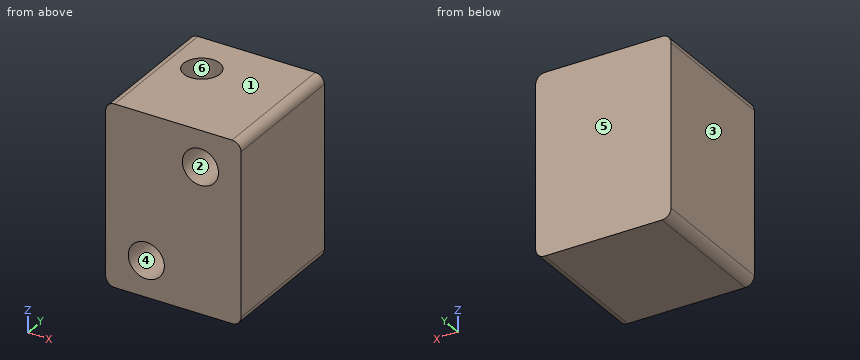
```python
from build123d import *

# Parameters (mm, degrees)
BOSS_EXTRU_1_DEPTH      = 15
ESQUISSE2_R             = 2
ENL_V_MAT_EXTRU_1_DEPTH = 12
ESQUISSE3_R             = 2
ENL_V_MAT_EXTRU_2_DEPTH = 12
CONG_1_R                = 1


with BuildPart() as part:
    # Esquisse1 → Boss.-Extru.1 (new body)
    with BuildSketch(Plane(origin=(0, 0, 0), x_dir=(1, 0, 0), z_dir=(0, 1, 0))):
        Polygon((0, 0), (7.5, 0), (7.5, 20), (-7.5, 20), (-7.5, 0), align=None)
    extrude(amount=BOSS_EXTRU_1_DEPTH)

    # Esquisse2 → Enlèv. mat.-Extru.1 (cut)
    with BuildSketch(Plane.XZ):
        with Locations(Location((-3, -16, 0), (0, 0, 270))):
            Circle(ESQUISSE2_R)
        with Locations(Location((3, -4, 0), (0, 0, 270))):
            Circle(ESQUISSE2_R)
    extrude(amount=-ENL_V_MAT_EXTRU_1_DEPTH, mode=Mode.SUBTRACT)

    # Esquisse3 → Enlèv. mat.-Extru.2 (cut)
    with BuildSketch(Plane.XY):
        with Locations((-3, 10)):
            Circle(ESQUISSE3_R)
    extrude(amount=-ENL_V_MAT_EXTRU_2_DEPTH, mode=Mode.SUBTRACT)

    # Congé1
    cong_1_edges = [part.edges().sort_by_distance(p)[0] for p in [
        (-7.5, 7.5, 0),
        (-7.5, 7.5, -20),
        (7.5, 7.5, -20),
        (7.5, 7.5, 0),
    ]]
    fillet(cong_1_edges, radius=CONG_1_R)


solid = part.part
```
Part model, mm, in its own coordinate system. Face numbers are marked on the shaded views. A direction names the side the tool comes from. Round coordinates to 2 decimals unless told otherwise and drop trailing zeros. Order: outer loops, then holes, each group sorted by start corner. A loop starts at its lowest first (then second) coordinate and runs counter-clockwise, first axis right, second up. Notation, with made-up numbers: M 53,15.25 L 61,15.25 A29 cw 61,50.25 Z; hole C 58,88 d7. An arc over 180 degrees is marked long. Put each result on its own line as item: value. Start each with the question number.
1. Drill centre lines: probe 1 along Y at (x, z) = (-3, -8.75); probe 2 along X at (y, z) = (9.75, -5.75); probe 3 along X at (y, z) = (7.5, -4). Where is each one in solid material? Low to high. Write a range as [from, to].
2. Slice it at D-D on y = 3.75. List the corners of the cut face in (x, z).
3. Slice it at C-C on z = -6.25. List the corners of the cut face in (x, y).
4. Drop flat-ended pins along their axis: pin 1 (2 mm diameter, centred on x = -5.5, z = -17, fed in from -Y); pin 2 (3 mm diameter, centred on x = 3, z = -4, fed in from -Y). Give the stop position or say it passes through.
5. Slice it at A-A on y = 10. List the corners of the cut face in (x, z).
6. Slice it at B-B on z = -16. List the corners of the cut face in (x, y), then the cut area to 3 significant figures.
7. Two-plate mould, pull along X, no slides. Class the marked faces 1, 2 and 3: +X half, -X half, draft (parallel to the pull), parting line (faces both ways), or undercut.
8. Tool access for the marked faces 4, 5 and 6: list every direction of +Z, -Z, +X, -X, +Y, -Y with a clear straight run to the whole face (end or side of a thin tool).
Findings:
1. probe 1: [0, 8], [12, 15]
1. probe 2: [-7.5, -4.98], [-1.02, 2.03], [3.97, 7.5]
1. probe 3: [-7.5, 1], [5, 7.5]
2. outline: M -7.5,-19 A1 ccw -6.5,-20 L 6.5,-20 A1 ccw 7.5,-19 L 7.5,-1 A1 ccw 6.5,0 L -6.5,0 A1 ccw -7.5,-1 Z; hole C -3,-16 d4; hole C 3,-4 d4
3. outline: M -7.5,0 L 7.5,0 L 7.5,15 L -7.5,15 Z; hole C -3,10 d4
4. pin 1: y = 0
4. pin 2: y = 12
5. outline: M -7.5,-19 A1 ccw -6.5,-20 L 6.5,-20 A1 ccw 7.5,-19 L 7.5,-1 A1 ccw 6.5,0 L -1,0 L -1,-12 L -5,-12 L -5,0 L -6.5,0 A1 ccw -7.5,-1 Z; hole C -3,-16 d4; hole C 3,-4 d4
6. outline: M -7.5,0 L -5,0 L -5,12 L -1,12 L -1,0 L 7.5,0 L 7.5,15 L -7.5,15 Z
6. area: 177 mm2
7. face 1: draft
7. face 2: undercut
7. face 3: -X half
8. face 4: -Y
8. face 5: +Z, -Z, +X, -X, +Y
8. face 6: +Z
